Build history of the part. All positions in model axes, mm. A direction names the side the tool comes from. Round coordinates to 2 decimals unless told otherwise and drop trailing zeros. Write each loop counter-clockwise with the first axis right and the second up, starting at its lowest first coordinate (ties: lowest second). Pieces come first, ordered by that corner, then holes.
Item 1: Wall check: probe 1 along X at (y, z) = (47, -54); probe 2 along X at (y, z) = (14.5, 0); probe 3 along X at (y, z) = (69, -231). Give the ranges that are in metal, low to high.
Item 2: Band-saw the part on C-C, the plane y = 70. Write the cut outline in (x, z), then the cut area to 3 significant figures.
Item 3: Mould opens along Z. For faces 1 (the cylindrical face through (102.83, 91.44, -232.86)), 2 (the cylindrical face through (78.1, 13.28, 17.34)), 3 (the flat face through (75.04, 58.95, -219.82)) say: +Z half, -Z half, draft (parallel to the pull), parting line (faces both ways), or undercut.
Item 4: Drop flat-ended pins along their axis: pin 1 Ø4 at (y, z) = (33.5, 34.5) entering from -X; pin 2 Ø8 at (x, y) = (180, 46) entering from -Z; pin 3 Ø5 at (x, z) = (139, 217) entering from -Y. Give the stop position or say it passes through.
Item 5: 3-axis set-ups, long thin cutter, end or side, ignore diameter. For faces 4 (the flat face through (-71.5, 36.2, -23.3)), 5 (the flat face through (101, 78, -243)), 6 (the flat face through (113.5, 55, -223)): which of +Z, -Z, +X, -X, +Y, -Y reach the whole face in a straight line?
Item 6: Band-saw the part on A-A, the plane y = 24. Write the cut outline in (x, z), then the cut area to 3 significant figures.
Item 7: Band-saw the part on D-D, the plane x = -37.5. Write the cut outline in (y, z), then the cut area to 3 significant figures.
Item 8: Band-saw the part on B-B, the plane x = 183. Write the cut outline in (y, z), then the cut area to 3 significant figures.
```python
from build123d import *

# Parameters (mm, degrees)
SKETCH_1_R          = 305
EXTRUDE_1_DEPTH     = 41.2
SKETCH_2_W          = 140
SKETCH_2_H          = 140
EXTRUDE_2_DEPTH     = 10
SHELL_1_T           = -5
CUT_EXTRUDE_1_DEPTH = 10
SKETCH_4_W          = 120
SKETCH_4_H          = 10
EXTRUDE_3_DEPTH     = 150
CUT_EXTRUDE_3_DEPTH = 648.322516216
SKETCH_6_R          = 10
CUT_EXTRUDE_5_DEPTH = 634.476787262
EXTRUDE_START       = 10
SKETCH_7_R          = 20
SKETCH_7_R_2        = 10
EXTRUDE_4_DEPTH     = 10
SKETCH_8_W          = 5
SKETCH_8_H          = 36
EXTRUDE_5_DEPTH     = 26
CUT_EXTRUDE_6_DEPTH = 536.715493522
SKETCH_10_W         = 5
SKETCH_10_H         = 46.5
SKETCH_10_W_2       = 19
SKETCH_10_H_2       = 5
SKETCH_11_R         = 8
SKETCH_11_R_2       = 4
CUT_EXTRUDE_7_DEPTH = 440.824965185


with BuildPart() as part:
    # 草图1 → 凸台-拉伸1 (new body)
    with BuildSketch(Plane(origin=(0, 0, 0), x_dir=(1, 0, 0), z_dir=(0, 1, 0))):
        with Locations(Location((0, 0, 0), (0, 0, 90))):
            Circle(SKETCH_1_R)
    extrude(amount=EXTRUDE_1_DEPTH)

    # 草图2 → 凸台-拉伸2 (add)
    with BuildSketch(Plane(origin=(0, 41.2, 0), x_dir=(1, 0, 0), z_dir=(0, 1, 0))):
        with Locations((183, 0)):
            Rectangle(SKETCH_2_W, SKETCH_2_H)
    extrude(amount=EXTRUDE_2_DEPTH)

    # 抽壳1
    shell_1_openings = [part.faces().sort_by_distance(p)[0] for p in [
        (0, 0, 0),
    ]]
    offset(amount=SHELL_1_T, openings=shell_1_openings, kind=Kind.INTERSECTION)

    # 草图3 → 切除-拉伸1 (cut)
    with BuildSketch(Plane(origin=(0, 41.2, 0), x_dir=(1, 0, 0), z_dir=(0, 1, 0))):
        with BuildLine():
            Line((-164, -24), (-100, -24))
            ThreePointArc((-100, -24), (-82, -42), (-100, -60))
            Line((-100, -60), (-164, -60))
            ThreePointArc((-164, -60), (-182, -42), (-164, -24))
        make_face()
    extrude(amount=-CUT_EXTRUDE_1_DEPTH, mode=Mode.SUBTRACT)

    # 草图4 → 凸台-拉伸3 (add)
    with BuildSketch(Plane(origin=(0, 41.2, 0), x_dir=(1, 0, 0), z_dir=(0, 1, 0))):
        with Locations((99, 238)):
            Rectangle(SKETCH_4_W, SKETCH_4_H)
    extrude(amount=EXTRUDE_3_DEPTH)

    # 草图5 → 切除-拉伸3 (cut, through all)
    with BuildSketch(Plane.XY.offset(-233)):
        with BuildLine():
            Line((131, 41.2), (159, 41.2))
            Line((159, 41.2), (159, 191.2))
            Line((159, 191.2), (39, 191.2))
            Line((39, 191.2), (39, 41.2))
            ThreePointArc((39, 41.2), (54.112125435, 81.748594957), (74.310300259, 120.018669715))
            ThreePointArc((74.310300259, 120.018669715), (114.95864882, 135.795163154), (140.99801314, 100.821780537))
            ThreePointArc((140.99801314, 100.821780537), (138.32356193, 70.621084147), (131, 41.2))
        make_face()
    extrude(amount=-CUT_EXTRUDE_3_DEPTH, mode=Mode.SUBTRACT)

    # 草图6 → 切除-拉伸5 (cut, through all)
    with BuildSketch(Plane.XY.offset(-233)):
        with Locations((105, 101.2)):
            Circle(SKETCH_6_R)
    extrude(amount=-CUT_EXTRUDE_5_DEPTH, mode=Mode.SUBTRACT)

    # 草图7 → 凸台-拉伸4 (add)
    with BuildSketch(Plane.XY.offset(-233).offset(EXTRUDE_START)):
        with Locations(Location((105, 101.2, 0), (0, 0, 180))):
            Circle(SKETCH_7_R)
        with Locations((105, 101.2)):
            Circle(SKETCH_7_R_2, mode=Mode.SUBTRACT)
    extrude(amount=-EXTRUDE_4_DEPTH)

    # 草图8 → 凸台-拉伸5 (add)
    with BuildSketch(Plane.XY.offset(-233)):
        with Locations((75, 59.2)):
            Rectangle(SKETCH_8_W, SKETCH_8_H)
        with Locations((111, 59.2)):
            Rectangle(SKETCH_8_W, SKETCH_8_H)
    extrude(amount=EXTRUDE_5_DEPTH)

    # 草图9 → 切除-拉伸6 (cut, through all)
    with BuildSketch(Plane(origin=(113.5, 0, 0), x_dir=(0, 0, -1), z_dir=(1, 0, 0))):
        Polygon((207, 41.2), (233, 77.2), (207, 77.2), align=None)
    extrude(amount=-CUT_EXTRUDE_6_DEPTH, mode=Mode.SUBTRACT)

    # 草图10 → 旋转1 (revolve)
    with BuildSketch(Plane.XY, mode=Mode.PRIVATE) as revolve_1_sk:
        with Locations((-82.5, 12.95)):
            Rectangle(SKETCH_10_W, SKETCH_10_H)
        with Locations((-65.5, 33.7)):
            Rectangle(SKETCH_10_W_2, SKETCH_10_H_2)
    revolve(revolve_1_sk.sketch.rotate(Axis((0, 0, 0), (0, 1, 0)), 270), axis=Axis((0, 0, 0), (0, 1, 0)))

    # 草图11 → 切除-拉伸7 (cut, through all)
    with BuildSketch(Plane(origin=(0, 51.2, 0), x_dir=(1, 0, 0), z_dir=(0, 1, 0))):
        with Locations(Location((183, 0, 0), (0, 0, 270))):
            Circle(SKETCH_11_R)
        with Locations(Location((237, 54, 0), (0, 0, 270))):
            Circle(SKETCH_11_R_2)
        with Locations(Location((129, 54, 0), (0, 0, 270))):
            Circle(SKETCH_11_R_2)
        with Locations(Location((129, -54, 0), (0, 0, 270))):
            Circle(SKETCH_11_R_2)
        with Locations(Location((237, -54, 0), (0, 0, 270))):
            Circle(SKETCH_11_R_2)
    extrude(amount=-CUT_EXTRUDE_7_DEPTH, mode=Mode.SUBTRACT)


solid = part.part
```
Results:
1. probe 1: x = 113 to 125, 133 to 233, 241 to 253
1. probe 2: x = -305 to -300, -85 to -80, 80 to 85, 300 to 305
1. probe 3: x = 72.5 to 77.5, 108.5 to 113.5
2. outline: (49.11, -243) - (138.22, -243) - (138.22, -233) - (113.5, -233) - (113.5, -227.8) - (108.5, -227.8) - (108.5, -233) - (77.5, -233) - (77.5, -227.8) - (72.5, -227.8) - (72.5, -233) - (49.11, -233) - close
2. area: 943 mm2
3. face 1: draft
3. face 2: undercut
3. face 3: +Z half
4. pin 1: stops at x = -303.26
4. pin 2: stops at z = -70
4. pin 3: stops at y = 36.2
5. face 4: -Y
5. face 5: -Z, +X, -X, +Y
5. face 6: +X
6. outline: circle Ø610 at (0, 0); circle Ø170 at (0, 0); hole circle Ø600 at (0, 0); hole circle Ø160 at (0, 0)
6. area: 12,100 mm2
7. outline: (-10.3, -76.28) - (36.2, -76.28) - (36.2, -297.65) - (0, -297.65) - (0, -302.69) - (41.2, -302.69) - (41.2, 302.69) - (0, 302.69) - (0, 297.65) - (36.2, 297.65) - (36.2, 76.28) - (-10.3, 76.28) - (-10.3, 70.67) - (36.2, 70.67) - (36.2, 64.95) - (31.2, 64.95) - (31.2, 41.59) - (36.2, 41.59) - (36.2, -41.59) - (31.2, -41.59) - (31.2, -64.95) - (36.2, -64.95) - (36.2, -70.67) - (-10.3, -70.67) - close
7. area: 4,150 mm2
8. outline: (0, -244) - (41.2, -244) - (41.2, -70) - (51.2, -70) - (51.2, -8) - (46.2, -8) - (46.2, -65) - (36.2, -65) - (36.2, -237.72) - (0, -237.72) - close; (0, 237.72) - (36.2, 237.72) - (36.2, 65) - (46.2, 65) - (46.2, 8) - (51.2, 8) - (51.2, 70) - (41.2, 70) - (41.2, 244) - (0, 244) - close
8. area: 2,910 mm2
